Build history of the part. All positions in model axes, mm. A direction names the side the tool comes from. Give positions to 0.01 mm unless a question says otherwise; leave off trailing zeros. Order: outer loops, then holes, each group sorted by start corner. A loop starts at its lowest first (then second) coordinate and runs counter-clockwise, first axis right, second up. Notation, with made-up numbers: (16, -1) - (60, -1) arc R21 cw to (60, 30) - close; hole circle Ø3 at (-33, -22.5). An arc over 180 degrees is marked (long way). Use a Markdown table: item, result. Add a question column.
(1) Mould opens along Z. For faces 4 (the face through (0, 0, 0)), 5 (the face through (52.46, -4.88, 1.08)), 6 (the face through (54.014, -1.756, -2.986)) say: +Z half, -Z half, draft (parallel to the pull), parting line (faces both ways), or undercut.
(2) Which spindle directions (+Z, -Z, +X, -X, +Y, -Y) get a long thin tool onto all of the face, cutting with end or side? Do faces 1 (the face through (53, 0, 0)), 2 (the face through (24.904, -3.905, 0.867)), 3 (the face through (55, -2.2, -3.3)). Say none if no direction does.
(3) Slice it at A-A (z = 0). Write the cut outline in (x, y).
(4) Flat gauge pins, fed straight in: pin 1 (6 mm diameter, centred on x = 28.5, z = 1, fed in from -Y); pin 2 (6 mm diameter, centred on x = 46.5, y = -2.5, fed in from -Z); pin 3 (2 mm diameter, centred on x = 22.5, y = -2, fed in from -Z). Where does each tip first touch, or does it go through?
(5) Wall check: line 1 (X direction, y = 2, z = 0); line 2 (X direction, y = -3, z = -3.25); line 3 (Z direction, x = 14, y = -2). Give the ranges that are in metal, low to high.
(6) Slice it at B-B (x = 30.5). Write the cut outline in (y, z).
from build123d import *

# Parameters (mm, degrees)
CROQUIS1_R              = 4
SALIENTE_EXTRUIR1_DEPTH = 50
CROQUIS2_R              = 5
SALIENTE_EXTRUIR2_DEPTH = 5
CORTAR_EXTRUIR1_DEPTH   = 2
CHAFL_N1_SIZE           = 0.5


with BuildPart() as part:
    # Croquis1 → Saliente-Extruir1 (new body)
    with BuildSketch(Plane(origin=(0, 0, 0), x_dir=(0, 0, -1), z_dir=(1, 0, 0))):
        Circle(CROQUIS1_R)
    extrude(amount=SALIENTE_EXTRUIR1_DEPTH)

    # Croquis2 → Saliente-Extruir2 (add)
    with BuildSketch(Plane(origin=(50, 0, 0), x_dir=(0, 0, -1), z_dir=(1, 0, 0))):
        Circle(CROQUIS2_R)
    extrude(amount=SALIENTE_EXTRUIR2_DEPTH)

    # Croquis3 → Cortar-Extruir1 (cut)
    with BuildSketch(Plane(origin=(55, 0, 0), x_dir=(0, 0, -1), z_dir=(1, 0, 0))):
        Polygon((4, 0), (2, 3.464101615), (-2, 3.464101615), (-4, 0), (-2, -3.464101615), (2, -3.464101615), align=None)
    extrude(amount=-CORTAR_EXTRUIR1_DEPTH, mode=Mode.SUBTRACT)

    # Chaflán1
    chafl_n1_edges = [part.edges().sort_by_distance(p)[0] for p in [
        (0, 0, 4),
    ]]
    chamfer(chafl_n1_edges, length=CHAFL_N1_SIZE)


solid = part.part
Solution:
| question | item | result |
|---|---|---|
| 1 | face 4 | draft |
| 1 | face 5 | parting line |
| 1 | face 6 | undercut |
| 2 | face 1 | +X |
| 2 | face 2 | -X |
| 2 | face 3 | +Z, -Z, +X, +Y, -Y |
| 3 | outline | (0, -3.5) - (0.5, -4) - (50, -4) - (50, -5) - (55, -5) - (55, -3.46) - (53, -3.46) - (53, 3.46) - (55, 3.46) - (55, 5) - (50, 5) - (50, 4) - (0.5, 4) - (0, 3.5) - close |
| 4 | pin 1 | y = -4 |
| 4 | pin 2 | z = -4 |
| 4 | pin 3 | z = -3.87 |
| 5 | line 1 | 0 to 53 |
| 5 | line 2 | 50 to 55 |
| 5 | line 3 | -3.46 to 3.46 |
| 6 | outline | circle Ø8 at (0, 0) |
